Verification items for the finished model (mm, model axes). Round coordinates to 2 decimals unless told otherwise and drop trailing zeros. Write each loop counter-clockwise with the first axis right and the second up, starting at its lowest first coordinate (ties: lowest second). Pieces come first, ordered by that corner, then holes. Notation, with made-up numbers: (54.25, -8) - (107.25, -8) arc R35 cw to (107.25, 24) - close; hole circle Ø7 at (18, 1). An arc over 180 degrees is marked (long way). Answer as a JSON object with one key per item and string values.
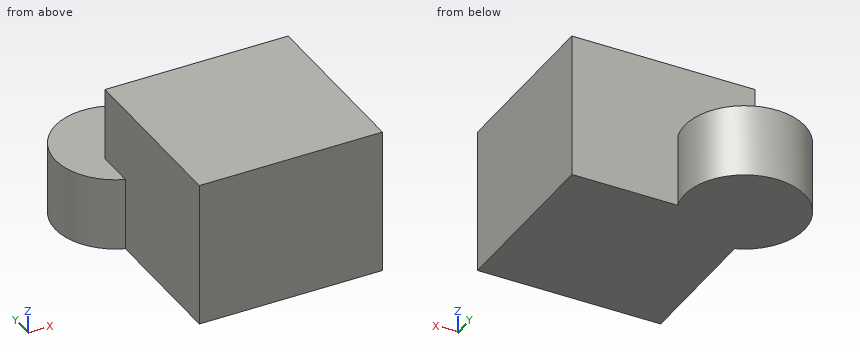
```python
from build123d import *

# Parameters (mm, degrees)
F0_W      = 63.8971067965
F0_H      = 61.4244844764
F1_DEPTH  = 25.4
F2_R      = 20.9044969904
F1_FACE_W = 63.8971067965
F1_FACE_H = 61.4244844764
F3_DEPTH  = 25.4


# Not quite as in the source:
# - a feature of the source that left no trace in its solid (it failed there, or was rolled back) is left out


with BuildPart() as f1:
    # F0 (on Top) → F1 (new body)
    with BuildSketch(Plane.XY):
        with Locations((-7.7395718545, 2.0738141611)):
            Rectangle(F0_W, F0_H)
    extrude(amount=F1_DEPTH)

    # F2 (on Top) + F1_face (on face) → F3 (join)
    with BuildSketch(Plane.XY):
        with Locations((-32.6551906765, 39.2090491951)):
            Circle(F2_R)
    with BuildSketch(Plane(origin=(-7.7395718545, 2.0738141611, 25.4), x_dir=(1, 0, 0), z_dir=(0, 0, 1))):
        Rectangle(F1_FACE_W, F1_FACE_H)
    extrude(amount=F3_DEPTH)


solid = f1.part
```
Q1. Section check D-D, the plane y = 29. Record the cut outline in (x, z), then the cut area to 3 significant figures.
Geometry check:
{"outline": "(-50.9, 0) - (24.21, 0) - (24.21, 50.8) - (-39.69, 50.8) - (-39.69, 25.4) - (-50.9, 25.4) - close", "area": "3,530 mm2"}
Q2. Section check C-C, the plane x = 1. Record the cut outline in (y, z), then the cut area to 3 significant figures.
Geometry check:
{"outline": "(-28.64, 0) - (32.79, 0) - (32.79, 50.8) - (-28.64, 50.8) - close", "area": "3,120 mm2"}
Q3. Gauge pin test, flat ends, axial feed: P1, Ø1, axis at y = 26, z = 15, coming from the -X side; P2, Ø15, axis at y = 2, z = 20, coming from the -X side; P3, Ø3, axis at x = -17.5, z = 6.5, coming from the +Y side. Record the tip position at first contact, or that the pin passes through.
Geometry check:
{"P1": "stops at x = -49.25", "P2": "stops at x = -39.69", "P3": "stops at y = 55.04"}
Q4. Section check B-B, the plane y = -13. Record the cut outline in (x, z).
Geometry check:
{"outline": "(-39.69, 0) - (24.21, 0) - (24.21, 50.8) - (-39.69, 50.8) - close"}
Q5. Section check A-A, the plane z = 14. Record the cut outline in (x, y).
Geometry check:
{"outline": "(-39.69, -28.64) - (24.21, -28.64) - (24.21, 32.79) - (-12.76, 32.79) arc R20.9 ccw (long way) to (-39.69, 19.52) - close"}
Q6. Material ranges on line 1 along Y through (x, z) = (-9, 6); line 2 along X through (y, z) = (-14.5, 2); line 3 along Z through (x, y) = (-24.5, 53), recorded low to high. Write a range as [from, to].
Geometry check:
{"line 1": "y = [-28.64, 32.79]", "line 2": "x = [-39.69, 24.21]", "line 3": "z = [0, 25.4]"}
